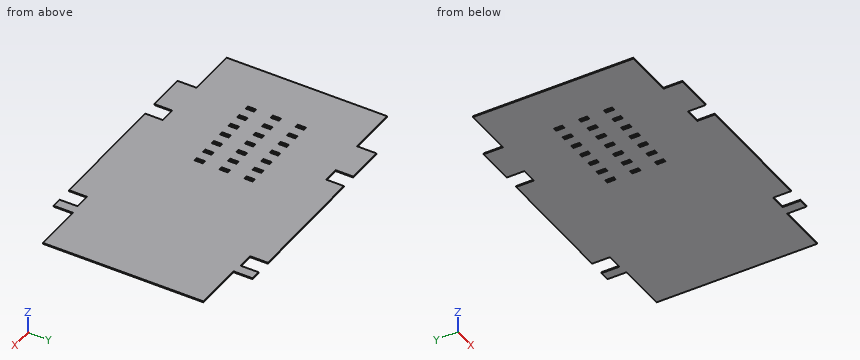
from build123d import *

# Parameters (mm, degrees)
F0_W     = 0.5
F0_H     = 1.2
F1_DEPTH = 0.15


with BuildPart() as f1:
    # F0 (on Top) → F1 (new body)
    with BuildSketch(Plane.XY):
        Polygon((25.1875, -11.3), (32.1875, -11.3), (32.1875, 11.3), (25.1875, 11.3), (25.1875, 14), (23.7875, 14), (23.7875, 11.5), (21.5875, 11.5), (21.5875, 14), (3.7875, 14), (3.7875, 11.5), (1.5875, 11.5), (1.5875, 14), (-3.8125, 14), (-3.8125, 11.3), (-10.8125, 11.3), (-10.8125, -11.3), (-3.8125, -11.3), (-3.8125, -14), (1.5875, -14), (1.5875, -11.5), (3.7875, -11.5), (3.7875, -14), (21.5875, -14), (21.5875, -11.5), (23.7875, -11.5), (23.7875, -14), (25.1875, -14), align=None)
        with Locations((-3.5625, -3.499541)):
            Rectangle(F0_W, F0_H, mode=Mode.SUBTRACT)
        with Locations((-1.5625, -3.499541)):
            Rectangle(F0_W, F0_H, mode=Mode.SUBTRACT)
        with Locations((0.4375, -3.499541)):
            Rectangle(F0_W, F0_H, mode=Mode.SUBTRACT)
        with Locations((2.4375, -3.499541)):
            Rectangle(F0_W, F0_H, mode=Mode.SUBTRACT)
        with Locations((4.4375, -3.499541)):
            Rectangle(F0_W, F0_H, mode=Mode.SUBTRACT)
        with Locations((6.4375, -3.499541)):
            Rectangle(F0_W, F0_H, mode=Mode.SUBTRACT)
        with Locations((8.4375, -3.499541)):
            Rectangle(F0_W, F0_H, mode=Mode.SUBTRACT)
        with Locations((-3.5625, 0.000459)):
            Rectangle(F0_W, F0_H, mode=Mode.SUBTRACT)
        with Locations((-1.5625, 0.000459)):
            Rectangle(F0_W, F0_H, mode=Mode.SUBTRACT)
        with Locations((-3.5625, 3.500459)):
            Rectangle(F0_W, F0_H, mode=Mode.SUBTRACT)
        with Locations((-1.5625, 3.500459)):
            Rectangle(F0_W, F0_H, mode=Mode.SUBTRACT)
        with Locations((0.4375, 0.000459)):
            Rectangle(F0_W, F0_H, mode=Mode.SUBTRACT)
        with Locations((2.4375, 0.000459)):
            Rectangle(F0_W, F0_H, mode=Mode.SUBTRACT)
        with Locations((4.4375, 0.000459)):
            Rectangle(F0_W, F0_H, mode=Mode.SUBTRACT)
        with Locations((6.4375, 0.000459)):
            Rectangle(F0_W, F0_H, mode=Mode.SUBTRACT)
        with Locations((8.4375, 0.000459)):
            Rectangle(F0_W, F0_H, mode=Mode.SUBTRACT)
        with Locations((0.4375, 3.500459)):
            Rectangle(F0_W, F0_H, mode=Mode.SUBTRACT)
        with Locations((2.4375, 3.500459)):
            Rectangle(F0_W, F0_H, mode=Mode.SUBTRACT)
        with Locations((4.4375, 3.500459)):
            Rectangle(F0_W, F0_H, mode=Mode.SUBTRACT)
        with Locations((6.4375, 3.500459)):
            Rectangle(F0_W, F0_H, mode=Mode.SUBTRACT)
        with Locations((8.4375, 3.500459)):
            Rectangle(F0_W, F0_H, mode=Mode.SUBTRACT)
    extrude(amount=F1_DEPTH)


solid = f1.part
CAD build for the part. Positions are in the model's coordinates, mm. Round coordinates to 2 decimals unless told otherwise and drop trailing zeros. Write each loop counter-clockwise with the first axis right and the second up, starting at its lowest first coordinate (ties: lowest second). Pieces come first, ordered by that corner, then holes. Notation, with made-up numbers: M -14,44 L 19,44 A22 ccw 19,71 Z; hole C 5,-24 d8. An arc over 180 degrees is marked long. Use a Markdown table: item, result. Add a question column.
1. Drill centre lines: probe 1 along X at (y, z) = (12.5, 0.05); probe 2 along Y at (x, z) = (23.5, 0.05). Where is each one in solid material? Low to high.
2. Slice it at A-A on y = 12. Give the cut face in (x, z), then the cut area to 3 significant figures.
3. Slice it at B-B on x = -7.5. Give the cut face in (y, z), then the cut area to 3 significant figures.
4. Slice it at D-D on x = 22. Give the cut face in (y, z).
5. Slice it at C-C on z = 0.1. Give the number of separate pieces and of enclosed holes in the cut face, then the cut area to 3 significant figures.
6. Flat gauge pin, fed straight in: P1, Ø2, axis at x = 12, y = 10, coming from the -Z side. Where does the tip first touch, or does it go through?
Reply:
| question | item | result |
|---|---|---|
| 1 | probe 1 | x = -3.81 to 1.59, 3.79 to 21.59, 23.79 to 25.19 |
| 1 | probe 2 | y = -11.5 to 11.5 |
| 2 | outline | M -3.81,0 L 1.59,0 L 1.59,0.15 L -3.81,0.15 Z; M 3.79,0 L 21.59,0 L 21.59,0.15 L 3.79,0.15 Z; M 23.79,0 L 25.19,0 L 25.19,0.15 L 23.79,0.15 Z |
| 2 | area | 3.69 mm^2 |
| 3 | outline | M -11.3,0 L 11.3,0 L 11.3,0.15 L -11.3,0.15 Z |
| 3 | area | 3.39 mm^2 |
| 4 | outline | M -11.5,0 L 11.5,0 L 11.5,0.15 L -11.5,0.15 Z |
| 5 | separate pieces | 1 |
| 5 | enclosed holes | 21 |
| 5 | area | 1,090 mm^2 |
| 6 | P1 | stops at z = 0 |
